Source: three-view drawing plus pictorial views. Frame: mm from the lowest corner of the part. A direction names the side the tool comes from. Give positions to 0.01 mm unless a question says otherwise; leave off trailing zeros. Write each loop counter-clockwise with the first axis right and the second up, starting at its lowest first coordinate (ties: lowest second). Pieces come first, ordered by that corner, then holes. Notation, with made-up numbers: (38, 89.5) - (89, 89.5) arc R20 ccw to (89, 96.5) - close; hole circle Ø3 at (61, 25). An arc over 180 degrees is marked (long way). One line per question, with ' | ' between items. Start each with the question number.
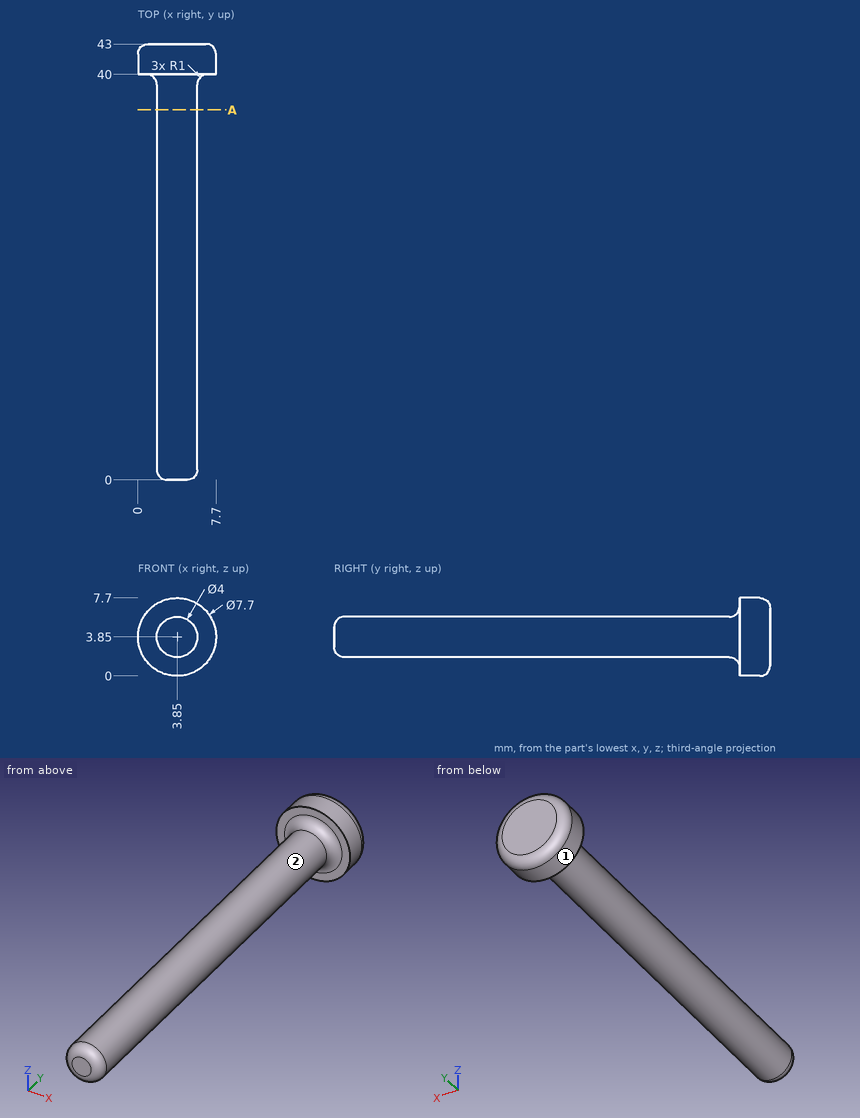
1) Reachability of the marked faces 1 and 2 from +Z, -Z, +X, -X, +Y, -Y: full face, straight path, thin tool, end or side. Return the list, or none.
2) Section A-A, the plane y = 36.5. Output: boundary loops of the cut face in (x, z), plus the area to 3 significant figures.
3) First-contact query: pin 1 Ø1 at (y, z) = (29.5, 3) entering from -X; pin 2 Ø1 at (y, z) = (28, 3) entering from +X; pin 3 Ø3 at (x, y) = (1, 34) entering from -Z. Flat tips, straight axial feed; report the tip coordinate or a pass-through.
4) Line query: L1, parallel to Y at x = 6.5, z = 2.5; L2, parallel to Z at x = 4.25, y = 10.5; L3, parallel to X at y = 30, z = 3.75. Output: solid intervals per line, ascending.
Answer key:
1) face 1: +Y, -Y | face 2: -Y
2) outline: circle Ø4 at (3.85, 3.85) | area: 12.6 mm^2
3) pin 1: x = 1.88 | pin 2: x = 5.82 | pin 3: z = 2.37
4) L1: 40 to 42.99 | L2: 1.89 to 5.81 | L3: 1.85 to 5.85
